Check sheet for the modelled part. Datum: model origin and axes. Units: mm. A direction names the side the tool comes from. Give positions to 0.01 mm unless a question says otherwise; leave off trailing zeros. Order: outer loops, then holes, each group sorted by start corner. A loop starts at its lowest first (then second) coordinate and runs counter-clockwise, first axis right, second up. Notation, with made-up numbers: (52.25, 32.25) -> (102.25, 32.25) arc R20 cw to (102.25, 44.25) -> close; hole circle Ø9 at (25, -12). An arc over 180 degrees is marked (long way). Write each question's results on one line, items separated by ' | '.
from build123d import *

# Parameters (mm, degrees)
SKETCH_1_W               = 90
SKETCH_1_H               = 90.00000171
SKETCH_1_R               = 12.5
SKETCH_1_R_2             = 1.5
EXTRUDE_1_DEPTH          = 5
CHAMFER_1_SIZE           = 5
SKETCH_2_R               = 34
SKETCH_2_R_2             = 31
EXTRUDE_2_DEPTH          = 3
EXTRUDE_3_DEPTH          = 42
CHAMFER_2_SIZE           = 5
SKETCH_4_W               = 15
SKETCH_4_H               = 25
CUT_EXTRUDE_1_DEPTH      = 157
PATTERN_CIRCULAR_1_COUNT = 2
PATTERN_CIRCULAR_1_ANGLE = 90
SKETCH_5_R               = 1.5
EXTRUDE_4_DEPTH          = 3


with BuildPart() as part:
    # 草图1 → 凸台-拉伸1 (new body)
    with BuildSketch(Plane(origin=(0, 0, 0), x_dir=(1, 0, 0), z_dir=(0, 1, 0))):
        Rectangle(SKETCH_1_W, SKETCH_1_H)
        with Locations(Location((0, 0, 0), (0, 0, 270))):
            Circle(SKETCH_1_R, mode=Mode.SUBTRACT)
        with Locations(Location((15.5, 15.500000294, 0), (0, 0, 270))):
            Circle(SKETCH_1_R_2, mode=Mode.SUBTRACT)
        with Locations(Location((-15.500000589, -15.499999706, 0), (0, 0, 90))):
            Circle(SKETCH_1_R_2, mode=Mode.SUBTRACT)
        with Locations(Location((15.500000589, -15.499999706, 0), (0, 0, 270))):
            Circle(SKETCH_1_R_2, mode=Mode.SUBTRACT)
        with Locations(Location((-15.5, 15.500000294, 0), (0, 0, 90))):
            Circle(SKETCH_1_R_2, mode=Mode.SUBTRACT)
    extrude(amount=EXTRUDE_1_DEPTH)

    # 倒角1
    chamfer_1_edges = [part.edges().sort_by_distance(p)[0] for p in [
        (45, 2.5, 45.000000855),
        (-45, 2.5, 45.000000855),
        (-45, 2.5, -45.000000855),
        (45, 2.5, -45.000000855),
    ]]
    chamfer(chamfer_1_edges, length=CHAMFER_1_SIZE)

    # 草图2 → 凸台-拉伸2 (add)
    with BuildSketch(Plane(origin=(0, 5, 0), x_dir=(1, 0, 0), z_dir=(0, 1, 0))):
        with Locations(Location((0, 0, 0), (0, 0, 90))):
            Circle(SKETCH_2_R)
        with Locations(Location((0, 0, 0), (0, 0, 270))):
            Circle(SKETCH_2_R_2, mode=Mode.SUBTRACT)
    extrude(amount=EXTRUDE_2_DEPTH)

    # 草图3 → 凸台-拉伸3 (add)
    # profile 1 of 4: a face of its own
    with BuildSketch(Plane.XZ):
        Polygon((25, 45.000000855), (40, 45.000000855), (45, 40.000000855), (45, 25.000000855), (30, 25.000000855), (25, 30.000000855), align=None)
        Polygon((28, 31.242641542), (31.242640687, 28.000000855), (42, 28.000000855), (42, 38.757360167), (38.757359313, 42.000000855), (28, 42.000000855), align=None, mode=Mode.SUBTRACT)
    # profile 2 of 4: a face of its own
    with BuildSketch(Plane.XZ):
        Polygon((25, -45.000000855), (25, -30.000000855), (30, -25.000000855), (45, -25.000000855), (45, -40.000000855), (40, -45.000000855), align=None)
        Polygon((28, -42.000000855), (28, -31.242641542), (31.242640687, -28.000000855), (42, -28.000000855), (42, -38.757360167), (38.757359313, -42.000000855), align=None, mode=Mode.SUBTRACT)
    # profile 3 of 4: a face of its own
    with BuildSketch(Plane.XZ):
        Polygon((-25, -45.000000855), (-40, -45.000000855), (-45, -40.000000855), (-45, -25.000000855), (-30, -25.000000855), (-25, -30.000000855), align=None)
        Polygon((-28, -42.000000855), (-38.757359313, -42.000000855), (-42, -38.757360167), (-42, -28.000000855), (-31.242640687, -28.000000855), (-28, -31.242641542), align=None, mode=Mode.SUBTRACT)
    # profile 4 of 4: a face of its own
    with BuildSketch(Plane.XZ):
        Polygon((-25, 45.000000855), (-25, 30.000000855), (-30, 25.000000855), (-45, 25.000000855), (-45, 40.000000855), (-40, 45.000000855), align=None)
        Polygon((-28, 42.000000855), (-28, 31.242641542), (-31.242640687, 28.000000855), (-42, 28.000000855), (-42, 38.757360167), (-38.757359313, 42.000000855), align=None, mode=Mode.SUBTRACT)
    extrude(amount=EXTRUDE_3_DEPTH)

    # 倒角2
    chamfer_2_edges = [part.edges().sort_by_distance(p)[0] for p in [
        (37.5, 0, -25.000000855),
        (25, 0, -37.500000855),
        (-25, 0, -37.500000855),
        (-37.5, 0, -25.000000855),
        (-37.5, 0, 25.000000855),
        (-25, 0, 37.500000855),
        (25, 0, 37.500000855),
        (37.5, 0, 25.000000855),
    ]]
    chamfer(chamfer_2_edges, length=CHAMFER_2_SIZE)

    # 草图4 → 切除-拉伸1 (cut)
    with BuildSketch(Plane(origin=(-42.500000427, 0, 42.500000427), x_dir=(0.7071067811865456, 0, 0.7071067811865495), z_dir=(-0.7071067811865495, 0, 0.7071067811865456))):
        with Locations((0, -20)):
            Rectangle(SKETCH_4_W, SKETCH_4_H)
    cut_extrude_1 = extrude(amount=-CUT_EXTRUDE_1_DEPTH, mode=Mode.SUBTRACT)

    # 阵列(圆周)1: 切除-拉伸1 ×2 about axis
    pattern_circular_1_axis = Axis((0, 8, 0), (0, -1, 0))
    for i in range(1, PATTERN_CIRCULAR_1_COUNT):
        add(cut_extrude_1.rotate(pattern_circular_1_axis, i * PATTERN_CIRCULAR_1_ANGLE / (PATTERN_CIRCULAR_1_COUNT - 1)), mode=Mode.SUBTRACT)

    # 草图5 → 凸台-拉伸4 (add)
    # profile 1 of 4: a face of its own
    with BuildSketch(Plane.XZ.offset(42)):
        Polygon((-25, -45.000000855), (-25, -30.000000855), (-30, -25.000000855), (-45, -25.000000855), (-45, -40.000000855), (-40, -45.000000855), align=None)
        with Locations(Location((-35, -35.000000855, 0), (0, 0, 90))):
            Circle(SKETCH_5_R, mode=Mode.SUBTRACT)
    # profile 2 of 4: a face of its own
    with BuildSketch(Plane.XZ.offset(42)):
        Polygon((40, -45.000000855), (45, -40.000000855), (45, -25.000000855), (30, -25.000000855), (25, -30.000000855), (25, -45.000000855), align=None)
        with Locations(Location((35, -35.000000855, 0), (0, 0, 270))):
            Circle(SKETCH_5_R, mode=Mode.SUBTRACT)
    # profile 3 of 4: a face of its own
    with BuildSketch(Plane.XZ.offset(42)):
        Polygon((25, 45.000000855), (25, 30.000000855), (30, 25.000000855), (45, 25.000000855), (45, 40.000000855), (40, 45.000000855), align=None)
        with Locations(Location((35, 35.000000855, 0), (0, 0, 90))):
            Circle(SKETCH_5_R, mode=Mode.SUBTRACT)
    # profile 4 of 4: a face of its own
    with BuildSketch(Plane.XZ.offset(42)):
        Polygon((-40, 45.000000855), (-45, 40.000000855), (-45, 25.000000855), (-30, 25.000000855), (-25, 30.000000855), (-25, 45.000000855), align=None)
        with Locations(Location((-35, 35.000000855, 0), (0, 0, 270))):
            Circle(SKETCH_5_R, mode=Mode.SUBTRACT)
    extrude(amount=-EXTRUDE_4_DEPTH)


solid = part.part
1. Section check C-C on z = 0.5. Record the cut outline in (x, y).
Verdict:
outline: (-45, 0) -> (-12.49, 0) -> (-12.49, 5) -> (-31, 5) -> (-31, 8) -> (-34, 8) -> (-34, 5) -> (-45, 5) -> close; (12.49, 0) -> (45, 0) -> (45, 5) -> (34, 5) -> (34, 8) -> (31, 8) -> (31, 5) -> (12.49, 5) -> close
2. Section check B-B on y = -34.5. Give the number of separate pieces and of enclosed holes in the cut face, then the cut area to 3 significant figures.
Verdict:
separate pieces: 4 | enclosed holes: 4 | area: 758 mm^2
3. Mould release check, pull along X, two halves, no side actions. Record for faces 6 (the flat face through (-1, 2, -45)), 7 (the flat face through (42, -19, 31)), 8 (the flat face through (43, -37, -42)), 9 (the flat face through (-43.521, -20.175, 32.914)): +X half, -X half, draft (parallel to the pull), parting line (faces both ways), or undercut.
Verdict:
face 6: draft | face 7: undercut | face 8: +X half | face 9: undercut
4. Gauge pin test, flat ends, axial feed: pin 1 Ø1.5 at (x, z) = (0.5, -35.5) entering from -Y; pin 2 Ø20 at (x, z) = (0, 0) entering from -Y; pin 3 Ø4 at (x, z) = (35, 34.5) entering from +Y. Record the tip position at first contact, or that the pin passes through.
Verdict:
pin 1: stops at y = 0 | pin 2: passes through | pin 3: stops at y = 5
5. Material ranges on probe 1 along X at (y, z) = (2, 15.5); probe 2 along X at (y, z) = (-39.9, 35); probe 3 along Z at (x, y) = (15, 1), recorded low to high. Write a range as from..to.
Verdict:
probe 1: x = -45..-17, -14..14, 17..45 | probe 2: x = -45..-36.5, -33.5..-25, 25..33.5, 36.5..45 | probe 3: z = -45..-16.91, -14.09..14.09, 16.91..45
6. Section check D-D on x = -15.5. Record the cut outline in (y, z).
Verdict:
outline: (0, -45) -> (5, -45) -> (5, -30.26) -> (8, -30.26) -> (8, -26.85) -> (5, -26.85) -> (5, -17) -> (0, -17) -> close; (0, -14) -> (5, -14) -> (5, 14) -> (0, 14) -> close; (0, 17) -> (5, 17) -> (5, 26.85) -> (8, 26.85) -> (8, 30.26) -> (5, 30.26) -> (5, 45) -> (0, 45) -> close
7. Access from +Z, -Z, +X, -X, +Y, -Y to the whole of each face (thin tool, end or side, straight path). Record for faces 1 (the flat face through (31, -19, -42)), 2 (the flat face through (26.479, -20.175, 37.086)), 3 (the cylindrical face through (-35.9, -40.5, 36.2)), 4 (the flat face through (-39, -3, 23)), 5 (the flat face through (-37.128, -20.175, -26.521)).
Verdict:
face 1: none | face 2: +X | face 3: -Y | face 4: +X, -X, -Y | face 5: -Z
8. Section check A-A on x = 0. Record the cut outline in (y, z).
Verdict:
outline: (0, -45) -> (5, -45) -> (5, -34) -> (8, -34) -> (8, -31) -> (5, -31) -> (5, -12.5) -> (0, -12.5) -> close; (0, 12.5) -> (5, 12.5) -> (5, 31) -> (8, 31) -> (8, 34) -> (5, 34) -> (5, 45) -> (0, 45) -> close
